from build123d import *

# Parameters (mm, degrees)
F3_DEPTH  = 7.62
F4_R      = 1.27
F5_R      = 1.27
F6_R      = 1.27
F7_R      = 1.27
F8_R      = 38.1635
F8_R_2    = 38.1
F8_R_3    = 6.35
F9_DEPTH  = 1.27
F10_R     = 6.35
F11_DEPTH = 1.27
F12_DEPTH = 5.08
F13_SIZE  = 1.27
F15_DEPTH = 5.08
F16_W     = 1.5503317118
F16_H     = 5.6140748784
F17_DEPTH = 12.7
F18_W     = 4.2479932308
F18_H     = 18.4551104903
F19_DEPTH = 25.4
F20_R     = 1.27
F21_W     = 1.4739185572
F21_H     = 3.6392435431
F22_DEPTH = 25.4
F24_W     = 19.498936832
F24_H     = 3.6067618057
F24_W_2   = 8.9468471706
F24_H_2   = 9.674844332
F25_DEPTH = 10.16
F23_R     = 3.3503869352
F26_DEPTH = 25.4
F27_R     = 2.54
F29_START = -7.62
F29_DEPTH = 2.54


with BuildPart() as f1:
    # F0 (on Front) → F1 (revolve)
    with BuildSketch(Plane.XZ):
        with BuildLine():
            Line((38.1, 5.1619349979), (38.1, 10.4672089629))
            Line((38.1, 10.4672089629), (35.3847315665, 12.8019368276))
            Line((35.3847315665, 12.8019368276), (0, 12.8019368276))
            Line((0, 12.8019368276), (0, -5.1619349979))
            Line((0, -5.1619349979), (0, -10.4672075979))
            Line((0, -10.4672075979), (38.1, -10.4672075979))
            Line((38.1, -10.4672075979), (38.1, -5.1619349979))
            ThreePointArc((38.1, -5.1619349979), (36.5098316879, 0), (38.1, 5.1619349979))
        make_face()
    revolve(axis=Axis((0, 0, 4.0121143684), (0, 0, -1)))

    # F2 (on face) → F3 (cut)
    with BuildSketch(Plane.XY.offset(12.8019368276)):
        with BuildLine():
            ThreePointArc((-4.5847, 8.3490209552), (0, 9.525), (4.5847, 8.3490209552))
            Line((4.5847, 8.3490209552), (14.9703790496, 24.6512715679))
            ThreePointArc((14.9703790496, 24.6512715679), (0.001087062, 28.3641023084), (-14.9668170137, 24.6456802915))
            Line((-14.9668170137, 24.6456802915), (-4.5847, 8.3490209552))
        make_face()
        with BuildLine():
            ThreePointArc((-8.72425296, -3.8227), (-9.525, 0), (-8.72425296, 3.8227))
            Line((-8.72425296, 3.8227), (-23.5637737238, 16.2087537647))
            ThreePointArc((-23.5637737238, 16.2087537647), (-27.8603099247, 2.364948039), (-26.2212824078, -12.0373007123))
            Line((-26.2212824078, -12.0373007123), (-8.72425296, -3.8227))
        make_face()
        with BuildLine():
            Line((14.9703790496, -24.6512715679), (4.5847, -8.3490209552))
            ThreePointArc((4.5847, -8.3490209552), (0, -9.525), (-4.5847, -8.3490209552))
            Line((-4.5847, -8.3490209552), (-14.9668170137, -24.6456802915))
            ThreePointArc((-14.9668170137, -24.6456802915), (0.001087062, -28.3641023084), (14.9703790496, -24.6512715679))
        make_face()
        with BuildLine():
            ThreePointArc((8.72425296, 3.8227), (9.3226641698, 1.9528332694), (9.525, 0))
            ThreePointArc((9.525, 0), (9.3226641698, -1.9528332694), (8.72425296, -3.8227))
            Line((8.72425296, -3.8227), (26.2212824078, -12.0373007123))
            ThreePointArc((26.2212824078, -12.0373007123), (27.8603099247, 2.364948039), (23.5637737238, 16.2087537647))
            Line((23.5637737238, 16.2087537647), (8.72425296, 3.8227))
        make_face()
    extrude(amount=-F3_DEPTH, mode=Mode.SUBTRACT)

    # F4
    f4_edges = [f1.edges().sort_by_distance(p)[0] for p in [
        (-23.563774, 16.208754, 8.991937),
        (-26.221282, -12.037301, 8.991937),
    ]]
    fillet(f4_edges, radius=F4_R)

    # F5
    f5_edges = [f1.edges().sort_by_distance(p)[0] for p in [
        (23.563774, 16.208754, 8.991937),
        (26.221282, -12.037301, 8.991937),
    ]]
    fillet(f5_edges, radius=F5_R)

    # F6
    f6_edges = [f1.edges().sort_by_distance(p)[0] for p in [
        (14.970379, 24.651272, 8.991937),
        (-14.966817, 24.64568, 8.991937),
    ]]
    fillet(f6_edges, radius=F6_R)

    # F7
    f7_edges = [f1.edges().sort_by_distance(p)[0] for p in [
        (-14.966817, -24.64568, 8.991937),
        (14.970379, -24.651272, 8.991937),
    ]]
    fillet(f7_edges, radius=F7_R)

    # F8 (on face) → F9 (join)
    with BuildSketch(Plane(origin=(0, 0, -10.4672075979), x_dir=(1, 0, 0), z_dir=(0, 0, -1))):
        Circle(F8_R)
        Circle(F8_R_2, mode=Mode.SUBTRACT)
        Circle(F8_R_2)
        with BuildLine():
            ThreePointArc((15.2978791062, 11.3524180179), (18.0876628807, 5.9782063793), (19.05, 0))
            ThreePointArc((19.05, 0), (18.0876628807, -5.9782063793), (15.2978791062, -11.3524180179))
            ThreePointArc((15.2978791062, -11.3524180179), (16.1086926372, -12.4523988749), (16.3958752879, -13.7884013423))
            ThreePointArc((16.3958752879, -13.7884013423), (14.2228751508, -16.8556128602), (10.6086050519, -15.8227683688))
            ThreePointArc((10.6086050519, -15.8227683688), (-7.4998811913, -17.511547108), (-18.7725642667, -3.2393411142))
            ThreePointArc((-18.7725642667, -3.2393411142), (-22.3012, 0), (-18.7725642667, 3.2393411142))
            ThreePointArc((-18.7725642667, 3.2393411142), (-7.4998811913, 17.511547108), (10.6086050519, 15.8227683688))
            ThreePointArc((10.6086050519, 15.8227683688), (14.2228751508, 16.8556128602), (16.3958752879, 13.7884013423))
            ThreePointArc((16.3958752879, 13.7884013423), (16.1086926372, 12.4523988749), (15.2978791062, 11.3524180179))
        make_face(mode=Mode.SUBTRACT)
        with BuildLine():
            ThreePointArc((15.2978791062, -11.3524180179), (18.0876628807, -5.9782063793), (19.05, 0))
            ThreePointArc((19.05, 0), (18.0876628807, 5.9782063793), (15.2978791062, 11.3524180179))
            ThreePointArc((15.2978791062, 11.3524180179), (10.9013173721, 11.4351808465), (10.6086050519, 15.8227683688))
            ThreePointArc((10.6086050519, 15.8227683688), (-7.4998811913, 17.511547108), (-18.7725642667, 3.2393411142))
            ThreePointArc((-18.7725642667, 3.2393411142), (-16.6549738523, 2.1986703236), (-15.7988, 0))
            ThreePointArc((-15.7988, 0), (-16.6549738523, -2.1986703236), (-18.7725642667, -3.2393411142))
            ThreePointArc((-18.7725642667, -3.2393411142), (-7.4998811913, -17.511547108), (10.6086050519, -15.8227683688))
            ThreePointArc((10.6086050519, -15.8227683688), (10.9013173721, -11.4351808465), (15.2978791062, -11.3524180179))
        make_face()
        Circle(F8_R_3, mode=Mode.SUBTRACT)
        Circle(F8_R_3)
    extrude(amount=F9_DEPTH)

    # F10 (on face) → F11 (join)
    with BuildSketch(Plane(origin=(0, 0, -11.7372075979), x_dir=(1, 0, 0), z_dir=(0, 0, -1))):
        Circle(F10_R)
    extrude(amount=F11_DEPTH)

    # F12 (add): faces of the model
    f12_faces = [f1.faces().sort_by_distance(p)[0] for p in [
        (-19.05, 0, -10.4672075979),
        (13.1446752879, -13.7884013423, -10.4672075979),
        (13.1446752879, 13.7884013423, -10.4672075979),
    ]]
    extrude(f12_faces, amount=F12_DEPTH)

    # F13
    f13_edges = [f1.edges().sort_by_distance(p)[0] for p in [
        (-19.327436, 3.239341, -15.547208),
        (10.991471, -16.224385, -15.547208),
        (15.680746, 11.754034, -15.547208),
    ]]
    chamfer(f13_edges, length=F13_SIZE)

    # F14 (on face) → F15 (cut)
    with BuildSketch(Plane(origin=(0, 0, -15.5472075979), x_dir=(1, 0, 0), z_dir=(0, 0, -1))):
        Polygon((-19.5883781174, -0.932498253), (-18.5116218826, -0.932498253), (-17.9732437653, 0), (-18.5116218826, 0.932498253), (-19.5883781174, 0.932498253), (-20.1267562347, 0), align=None)
        Polygon((12.6079911033, 12.7593241632), (13.7598334213, 12.7593241632), (14.3357545803, 13.7568488717), (13.7598334213, 14.7543735802), (12.6079911033, 14.7543735802), (12.0320699444, 13.7568488717), align=None)
        Polygon((13.7116949347, -12.7356480807), (12.3682391557, -12.7356480807), (11.6965112661, -13.8991149142), (12.3682391557, -15.0625817478), (13.7116949347, -15.0625817478), (14.3834228243, -13.8991149142), align=None)
    extrude(amount=-F15_DEPTH, mode=Mode.SUBTRACT)

    # F16 (on Front) → F17 (join, symmetric)
    with BuildSketch(Plane.XZ):
        Polygon((-32.2118215263, -11.686575599), (-32.2118215263, -10.4102920741), (-42.9334044456, -10.4102920741), (-42.9334044456, -11.686575599), (-41.3830727339, -11.686575599), align=None)
        with Locations((-42.1582385898, -14.4936130382)):
            Rectangle(F16_W, F16_H)
        Polygon((-41.3830727339, -17.3006504774), (-42.9334044456, -17.3006504774), (-51.4909774065, -17.3006504774), (-51.4909774065, -18.2480737567), (-41.3830727339, -18.2480737567), align=None)
    extrude(amount=F17_DEPTH, both=True)

    # F18 (on face) → F19 (cut)
    with BuildSketch(Plane.XY.offset(-17.3006504774)):
        with Locations((-47.2121909261, 0)):
            Rectangle(F18_W, F18_H)
    extrude(amount=-F19_DEPTH, mode=Mode.SUBTRACT)

    # F20
    f20_edges = [f1.edges().sort_by_distance(p)[0] for p in [
        (-49.336188, 9.227555, -17.774362),
        (-45.088194, 9.227555, -17.774362),
        (-49.336188, -9.227555, -17.774362),
        (-45.088194, -9.227555, -17.774362),
    ]]
    fillet(f20_edges, radius=F20_R)

    # F21 (on Front) → F22 (join, symmetric)
    with BuildSketch(Plane.XZ):
        Polygon((43.6872541904, -10.6276860461), (22.8208769113, -10.6276860461), (22.8208769113, -11.7372768), (42.2133356333, -11.7372768), (43.6872541904, -11.7372768), align=None)
        with Locations((42.9502949119, -13.5568985716)):
            Rectangle(F21_W, F21_H)
        Polygon((53.3728897572, -15.3765203431), (43.6872541904, -15.3765203431), (42.2133356333, -15.3765203431), (42.2133356333, -17.6648404449), (53.3728897572, -17.6648404449), align=None)
    extrude(amount=F22_DEPTH, both=True)

    # F24 (on Front) → F25 (cut, symmetric)
    with BuildSketch(Plane.XZ):
        Polygon((61.5164451301, -8.7059047073), (28.3735431731, -8.7059047073), (28.3735431731, -11.3572236151), (42.0175082982, -11.3572236151), (61.5164451301, -11.3572236151), align=None)
        with Locations((51.7669767141, -13.1606045179)):
            Rectangle(F24_W, F24_H)
        with Locations((65.9898687154, -19.8014075868)):
            Rectangle(F24_W_2, F24_H_2)
        with Locations((51.7669767141, -19.8014075868)):
            Rectangle(F24_W, F24_H_2)
    extrude(amount=F25_DEPTH, both=True, mode=Mode.SUBTRACT)

    # F23 (on face) → F26 (cut)
    with BuildSketch(Plane.XY.offset(-15.3765203431)):
        with Locations((49.1436608136, 18.2800516486)):
            Circle(F23_R)
        with Locations((49.1436608136, -18.2800516486)):
            Circle(F23_R)
    extrude(amount=-F26_DEPTH, mode=Mode.SUBTRACT)

    # F27
    f27_edges = [f1.edges().sort_by_distance(p)[0] for p in [
        (43.687254, 17.78, -10.627686),
        (42.213336, 17.78, -17.66484),
        (42.213336, -17.78, -17.66484),
        (43.687254, -17.78, -10.627686),
        (53.37289, -25.4, -16.52068),
        (53.37289, -10.16, -16.52068),
        (53.37289, 10.16, -16.52068),
        (53.37289, 25.4, -16.52068),
        (-42.933404, 0, -10.410292),
        (-41.383073, 0, -18.248074),
        (-51.490977, -12.7, -17.774362),
        (-51.490977, 12.7, -17.774362),
    ]]
    fillet(f27_edges, radius=F27_R)

    # F28 (on Top) → F29 (join)
    with BuildSketch(Plane.XY.offset(F29_START)):
        Polygon((-38.9726124704, 14.9672068655), (-31.745903194, 14.9672068655), (-26.2082958382, 25.8024390787), (-33.5525795817, 25.8024390787), (-38.9726124704, 21.4135237038), align=None)
        Polygon((-26.2082958382, -25.8024390787), (-31.745903194, -14.9672068655), (-38.9726124704, -14.9672068655), (-38.9726124704, -21.4135237038), (-33.5525795817, -25.8024390787), align=None)
    extrude(amount=-F29_DEPTH)


solid = f1.part
Part model, mm, in its own coordinate system. A direction names the side the tool comes from. Give positions to 0.01 mm unless a question says otherwise; leave off trailing zeros. Loops run counter-clockwise (first coordinate to the right, second up) from the corner with the lowest first, then second, coordinate; pieces in that order, holes last. Notation, with made-up numbers: (-13, -30) -> (-1, -30) arc R11 ccw to (-1, -20) -> close; hole circle Ø7 at (38, -12). An arc over 180 degrees is marked (long way). Write each question's results on one line, items separated by ' | '. Start each with the question number.
Q1. Pull direction Y, two halves, no side cores. Call faces 4 (the face through (-27.85, 2.49, 9.05)), 5 (the face through (-50.7, 12, -17.8)), 6 (the face through (-41.383, 0, -14)): +Y half, -Y half, draft (parallel to the pull), parting line (faces both ways), or undercut.
Q2. Band-saw the part on B-B on z = -2. List the corners of the cut face in (x, y).
Q3. Wall check: L1, parallel to Z at x = -29, y = -2; L2, parallel to Z at x = -37, y = -16; L3, parallel to X at y = 4, z = -16. Give the ranges that are in metal, low to high.
Q4. Pin check, flat tips, straight feed: P1, Ø5.5, axis at x = 49.14, y = 18.28, coming from the +Z side; P2, Ø0.5, axis at y = 2.5, z = -17.5, coming from the +X side; P3, Ø5, axis at y = 11.5, z = -15, coming from the -X side; P4, Ø0.8, axis at x = -37, z = -9, coming from the +Y side. Stop position of each tip, or through.
Q5. Which spindle directions (+Z, -Z, +X, -X, +Y, -Y) get a long thin tool onto all of the face, cutting with end or side? Do faces 1 (the face through (43, 25.4, -14)), 2 (the face through (46, 16, -15.377)), 3 (the face through (52.609, -10.884, -16.537)). Say none if no direction does.
Results are:
1) face 4: undercut | face 5: +Y half | face 6: draft
2) outline: circle Ø73.46 at (0, 0)
3) L1: z = -11.74 to 12.8 | L2: z = -10.16 to -7.62 | L3: x = -42.93 to -41.4
4) P1: passes through | P2: stops at x = -41.9 | P3: stops at x = -51.47 | P4: stops at y = 23.33
5) face 1: +Z, -Z, +X, +Y | face 2: +Z, +X, +Y, -Y | face 3: +Z, -Z, +X
